from build123d import *

# Parameters (mm, degrees)
F0_R     = 5
F1_DEPTH = 6
F2_R     = 3
F3_DEPTH = 40
F5_DEPTH = 3
F6_SIZE  = 0.6


with BuildPart() as f1:
    # F0 (on Front) → F1 (new body)
    with BuildSketch(Plane.XZ):
        Circle(F0_R)
    extrude(amount=F1_DEPTH)

    # F2 (on face) → F3 (join)
    with BuildSketch(Plane.XZ.offset(6)):
        Circle(F2_R)
    extrude(amount=F3_DEPTH)

    # F4 (on face) → F5 (cut)
    with BuildSketch(Plane(origin=(0, 0, 0), x_dir=(-1, 0, 0), z_dir=(0, 1, 0))):
        Polygon((1.443376, 2.5), (-1.443376, 2.5), (-2.886751, 0), (-1.443376, -2.5), (1.443376, -2.5), (2.886751, 0), align=None)
    extrude(amount=-F5_DEPTH, mode=Mode.SUBTRACT)

    # F6
    f6_edges = [f1.edges().sort_by_distance(p)[0] for p in [
        (-5, 0, 0),
        (-3, -46, 0),
    ]]
    chamfer(f6_edges, length=F6_SIZE)


solid = f1.part
The model under review builds one solid part; all positions refer to its coordinate system, in mm. A direction names the side the tool comes from. Round coordinates to 2 decimals unless told otherwise and drop trailing zeros. Write each loop counter-clockwise with the first axis right and the second up, starting at its lowest first coordinate (ties: lowest second). Pieces come first, ordered by that corner, then holes. Notation, with made-up numbers: M -11.75,13.25 L 46.25,13.25 A22 ccw 46.25,45.25 Z; hole C 15,58.25 d7. An arc over 180 degrees is marked long. Use a Markdown table: item, result. Add a question column.
Q1. The part is to be moulded in two halves that separate along X. For faces 4 (the face through (-3, -25, 0)), 5 (the face through (0, -1, -2.5)), 6 (the face through (0, -46, 0)), say which applies: pulls with the +X half, pulls with the -X half, needs draft (parallel to the pull), parting line crosses it, or undercut.
Q2. To check wall thickness, follow line 1 (Y direction, x = -0.5, z = 0.25); line 2 (Y direction, x = 4.25, z = -0.25); line 3 (X direction, y = -14.5, z = 1). State the ranges of each line that lie inside material, in increasing order.
Q3. We need section A-A, the plane x = 0. State the section outline as (y, z) points.
Q4. We need section B-B, the plane y = -28. State the section outline as (x, z) points.
Q5. Machinability: for faces 1 (the face through (-2.175, -1.479, 1.233)), 2 (the face through (-0.1, -6, -3.3)), 3 (the face through (-1.08, -3.26, -4.88)), which of the approach directions +Z, -Z, +X, -X, +Y, -Y give a long, thin tool a straight path to every point of the face, cutting with its end or side? Answer none if there is none.
Q6. Insertion check: pin 1 (1 mm diameter, centred on y = -16, z = 1, fed in from -X); pin 2 (4 mm diameter, centred on y = -5.5, z = -4, fed in from -X). Each pin has a flat end and moves straight along its axis. Give the tip position at first contact, or say it passes through.
Findings below:
| question | item | result |
|---|---|---|
| 1 | face 4 | parting line crosses it |
| 1 | face 5 | undercut |
| 1 | face 6 | needs draft |
| 2 | line 1 | y = -46 to -3 |
| 2 | line 2 | y = -6 to 0 |
| 2 | line 3 | x = -2.83 to 2.83 |
| 3 | outline | M -46,-2.4 L -45.4,-3 L -6,-3 L -6,-5 L -0.6,-5 L 0,-4.4 L 0,-2.5 L -3,-2.5 L -3,2.5 L 0,2.5 L 0,4.4 L -0.6,5 L -6,5 L -6,3 L -45.4,3 L -46,2.4 Z |
| 4 | outline | C 0,0 d6 |
| 5 | face 1 | +Y |
| 5 | face 2 | -Y |
| 5 | face 3 | +Y, -Y |
| 6 | pin 1 | stops at x = -2.96 |
| 6 | pin 2 | stops at x = -4.58 |
